```python
from build123d import *

# Parameters (mm, degrees)
SKETCH011_R             = 4
PAD004_DEPTH            = 1.5
SKETCH012_R             = 2
PAD005_DEPTH            = 6.3
SKETCH013_W             = 3
SKETCH013_H             = 4
POCKET004_DEPTH         = 1.1
FILLET004_R             = 1
SKETCH014_R             = 1.1
POCKET010_DEPTH         = 3
FILLET016_R             = 0.75
BODY002_PLACEMENT_ANGLE = 90


with BuildPart() as part:
    # Sketch011 → Pad004 (new body)
    with BuildSketch(Plane.XY):
        Polygon((29.8, 11.3), (24.8, 11.3), (24.8, 12.8), (15.2, 12.8), (15.2, 11.3), (-14.8, 11.3), (-14.8, -11.3), (15.2, -11.3), (15.2, -12.8), (24.8, -12.8), (24.8, -11.3), (29.8, -11.3), align=None)
        with Locations((-2.325, 1.95)):
            Circle(SKETCH011_R, mode=Mode.SUBTRACT)
    extrude(amount=PAD004_DEPTH)

    # Sketch012 → Pad005 (join)
    with BuildSketch(Plane.XY):
        with Locations((6.3, -7)):
            Circle(SKETCH012_R)
        with Locations((-7.7, -7)):
            Circle(SKETCH012_R)
    extrude(amount=-PAD005_DEPTH)

    # Sketch013 → Pocket004 (cut)
    with BuildSketch(Plane.XY):
        with Locations((-9.125, 1.95)):
            Rectangle(SKETCH013_W, SKETCH013_H)
    extrude(amount=POCKET004_DEPTH, mode=Mode.SUBTRACT)

    # Fillet004
    fillet004_edges = [part.edges().sort_by_distance(p)[0] for p in [
        (4.3, -7, 0),
        (-9.7, -7, 0),
    ]]
    fillet(fillet004_edges, radius=FILLET004_R)

    # Sketch014 → Pocket010 (cut)
    with BuildSketch(Plane.XY.offset(-6.3)):
        with Locations((-7.7, -7)):
            Circle(SKETCH014_R)
        with Locations((6.3, -7)):
            Circle(SKETCH014_R)
    extrude(amount=POCKET010_DEPTH, mode=Mode.SUBTRACT)

    # Fillet016
    fillet016_edges = [part.edges().sort_by_distance(p)[0] for p in [
        (27.3, -11.3, 1.5),
        (29.8, 0, 1.5),
        (27.3, 11.3, 1.5),
        (24.8, 12.05, 1.5),
        (20, 12.8, 1.5),
        (15.2, 12.05, 1.5),
        (0.2, 11.3, 1.5),
        (-14.8, 0, 1.5),
        (0.2, -11.3, 1.5),
        (15.2, -12.05, 1.5),
        (20, -12.8, 1.5),
        (24.8, -12.05, 1.5),
        (-6.325, 1.95, 1.5),
    ]]
    fillet(fillet016_edges, radius=FILLET016_R)


with BuildPart() as part_1:
    # Body002 placement: moved
    add(part.part.moved(Location((39, -34, 18.8))).rotate(Axis((39, -34, 18.8), (0, 0, 1)), BODY002_PLACEMENT_ANGLE))


solid = part_1.part
```
Can you work these out from the model? Positions are in its coordinate system, mm. A direction names the side the tool comes from. Coordinates: 2 decimals unless noted, no trailing zeros. Loops run counter-clockwise (first coordinate to the right, second up) from the corner with the lowest first, then second, coordinate; pieces in that order, holes last. Notation, with made-up numbers: (81, -37.75) - (85, -37.75) arc R20 ccw to (85, -9.75) - close; hole circle Ø6 at (7, -17.75). An arc over 180 degrees is marked (long way). Use a Markdown table: item, result.
Item 1: Will these pins go through, and if not, where does the flat tip stop? pin 1 (1.1 mm diameter, centred on x = 46, y = -41.5, fed in from -Z); pin 2 (1.5 mm diameter, centred on x = 43.5, y = -23, fed in from -Z); pin 3 (0.9 mm diameter, centred on x = 36, y = -44, fed in from -Z).
Numbers:
| item | result |
|---|---|
| pin 1 | stops at z = 15.5 |
| pin 2 | stops at z = 18.8 |
| pin 3 | stops at z = 19.9 |
Item 2: I want a section at B-B on z = 17. Please give me the cut outline in (x, y), and give its area (3 significant figures).
Numbers:
| item | result |
|---|---|
| outline | circle Ø4 at (46, -41.7); circle Ø4 at (46, -27.7) |
| area | 25.1 mm2 |
Item 3: I want a section at A-A on x = 37.05. Please give me the cut outline in (y, z) (3 decimals).
Numbers:
| item | result |
|---|---|
| outline | (-48.8, 18.8) - (-44.625, 18.8) - (-44.625, 19.9) - (-41.625, 19.9) - (-41.625, 18.8) - (-40.325, 18.8) - (-40.325, 19.55) arc R0.75 ccw to (-41.075, 20.3) - (-48.05, 20.3) arc R0.75 ccw to (-48.8, 19.55) - close; (-32.325, 18.8) - (-4.2, 18.8) - (-4.2, 19.55) arc R0.75 ccw to (-4.95, 20.3) - (-31.575, 20.3) arc R0.75 ccw to (-32.325, 19.55) - close |
Item 4: I want a section at D-D on y = -24. Please give me the cut outline in (x, z).
Numbers:
| item | result |
|---|---|
| outline | (27.7, 18.8) - (50.3, 18.8) - (50.3, 19.55) arc R0.75 ccw to (49.55, 20.3) - (28.45, 20.3) arc R0.75 ccw to (27.7, 19.55) - close |
Item 5: For faces 1 (the face through (47.952, -28.134, 15.187)), 2 (the face through (46.9, -26.8, 12.5)), which set-ups out of +Z, -Z, +X, -X, +Y, -Y let a thin tool reach every point of the face, with its end or its side?
Numbers:
| item | result |
|---|---|
| face 1 | -Z |
| face 2 | -Z, +X, -X, +Y, -Y |
Item 6: I want a section at C-C on x = 30.75. Please give me the cut outline in (y, z).
Numbers:
| item | result |
|---|---|
| outline | (-48.8, 18.8) - (-4.2, 18.8) - (-4.2, 19.55) arc R0.75 ccw to (-4.95, 20.3) - (-48.05, 20.3) arc R0.75 ccw to (-48.8, 19.55) - close |
Item 7: If I drill on probe 1 along Y at (x, z) = (46, 13.6); probe 2 along X at (y, z) = (-41.7, 14.6); probe 3 along Z at (x, y) = (48.5, -11.5), over which ranges is the centre line in solid material (lowest first)? Write a range as from..to.
Numbers:
| item | result |
|---|---|
| probe 1 | y = -43.7..-42.8, -40.6..-39.7, -29.7..-28.8, -26.6..-25.7 |
| probe 2 | x = 44..44.9, 47.1..48 |
| probe 3 | z = 18.8..20.3 |
Item 8: We'd pull the mould along Y, two halves only. Please class faces 3 (the face through (38.58, -32.63, 19.17)), 4 (the face through (46.9, -40.8, 12.5)): released by +Y, released by -Y, zero draft, split by the parting line, or undercut.
Numbers:
| item | result |
|---|---|
| face 3 | undercut |
| face 4 | zero draft |
